Verification items for the finished model (mm, model axes). A direction names the side the tool comes from. Round coordinates to 2 decimals unless told otherwise and drop trailing zeros. Write each loop counter-clockwise with the first axis right and the second up, starting at its lowest first coordinate (ties: lowest second). Pieces come first, ordered by that corner, then holes. Notation, with made-up numbers: M -37,86 L 11,86 A36 cw 11,125 Z; hole C -19,48.5 d8. An arc over 180 degrees is marked long. One line per question, with ' | ' between items.
from build123d import *

# Parameters (mm, degrees)
F1_DEPTH = 63.5
F2_DEPTH = 25.4
F3_DEPTH = 3.3655
F6_R     = 6.35
F7_R     = 2.54
F8_R     = 2.54


with BuildPart() as f1:
    # F0 (on Front) → F1 (new body, symmetric)
    with BuildSketch(Plane.XZ):
        Polygon((-41.275, -9.525), (41.275, -9.525), (41.275, 9.525), (22.225, 9.525), (-41.275, 9.525), align=None)
    extrude(amount=F1_DEPTH, both=True)

    # F0 (on Front) → F2 (join, symmetric)
    with BuildSketch(Plane.XZ):
        with BuildLine():
            Line((22.225, 9.525), (41.275, 9.525))
            Line((41.275, 9.525), (41.275, 27.305))
            ThreePointArc((41.275, 27.305), (45.9246798487, 38.5303201513), (57.15, 43.18))
            Line((57.15, 43.18), (64.7230581194, 43.18))
            Line((64.7230581194, 43.18), (64.7230581194, 62.23))
            Line((64.7230581194, 62.23), (57.15, 62.23))
            ThreePointArc((57.15, 62.23), (32.4542956671, 52.0007043329), (22.225, 27.305))
            Line((22.225, 27.305), (22.225, 9.525))
        make_face()
    extrude(amount=F2_DEPTH, both=True)

    # F0 (on Front) → F3 (join, symmetric)
    with BuildSketch(Plane.XZ):
        with BuildLine():
            add(Edge.make_bspline(
                [(-41.275, 9.525), (-13.7296449393, 37.2954718769), (24.3855025619, 65.1646107435), (64.7230581194, 62.23)],
                knots=[0, 0, 0, 0, 118.3782300514, 118.3782300514, 118.3782300514, 118.3782300514], degree=3))
            Line((-41.275, 9.525), (22.225, 9.525))
            Line((22.225, 9.525), (22.225, 27.305))
            ThreePointArc((22.225, 27.305), (32.4542956671, 52.0007043329), (57.15, 62.23))
            Line((57.15, 62.23), (64.7230581194, 62.23))
        make_face()
    extrude(amount=F3_DEPTH, both=True)

    # F0 (on Front) → F5 (revolve)
    with BuildSketch(Plane.XZ):
        Polygon((85.725, 66.675), (85.725, 62.23), (85.725, 43.18), (85.725, 38.1), (115.5230581194, 38.1), (115.5230581194, 66.675), align=None)
    revolve(axis=Axis((85.3036269546, 0, 52.5564104319), (0, 0, -1)))

    # F6
    f6_edges = [f1.edges().sort_by_distance(p)[0] for p in [
        (-41.275, -63.5, 0),
        (41.275, -63.5, 0),
        (41.275, 63.5, 0),
        (-41.275, 63.5, 0),
    ]]
    fillet(f6_edges, radius=F6_R)

    # F7
    f7_edges = [f1.edges().sort_by_distance(p)[0] for p in [
        (64.723058, -25.4, 52.705),
    ]]
    fillet(f7_edges, radius=F7_R)

    # F8
    f8_edges = [f1.edges().sort_by_distance(p)[0] for p in [
        (64.723058, 25.4, 52.705),
    ]]
    fillet(f8_edges, radius=F8_R)


solid = f1.part
1. Tool access check on faces 1 (the face through (86, 0, 38.1)), 2 (the face through (37, -25.4, 36)), 3 (the face through (37, 25.4, 36)). Record the directions out of +Z, -Z, +X, -X, +Y, -Y that give a thin tool (end or side, any length) a straight path to the whole face; none if there is none.
Results:
face 1: -Z, +X, +Y, -Y | face 2: +Z, -X, -Y | face 3: +Z, -X, +Y
2. Thickness scan on line 1 (Z direction, x = 9.5, y = -52) (3 decimals); line 2 (Y direction, x = -17, z = 27); line 3 (Z direction, x = 85, y = -4) (3 decimals). Record the ranges inside material, lowest first.
Results:
line 1: z = -9.525 to 9.525 | line 2: y = -3.37 to 3.37 | line 3: z = 38.1 to 66.675
3. Go/stop test with flat-tipped pins: P1, Ø2, axis at x = 43, y = 7.5, coming from the +Z side; P2, Ø4, axis at y = -0.5, z = 19, coming from the -X side; P3, Ø9, axis at y = -11, z = 14.5, coming from the -X side (3 decimals); P4, Ø6, axis at x = 50.5, y = 31, coming from the +Z side. Record where each tip stops, or that it passes through.
Results:
P1: stops at z = 59.66 | P2: stops at x = -33.59 | P3: stops at x = 22.225 | P4: passes through
4. Section check C-C, the plane x = 59. Record the cut outline in (y, z) (3 decimals).
Results:
outline: M -25.4,43.18 L -14.877,43.18 L -14.877,38.1 L 14.877,38.1 L 14.877,43.18 L 25.4,43.18 L 25.4,62.23 L 14.877,62.23 L 14.877,66.675 L -14.877,66.675 L -14.877,62.23 L -25.4,62.23 Z
5. Section check A-A, the plane z = 2.5. Record the cut outline in (x, y) (3 decimals), then the cut area to 3 significant figures.
Results:
outline: M -41.275,-57.15 A6.35 ccw -34.925,-63.5 L 34.925,-63.5 A6.35 ccw 41.275,-57.15 L 41.275,57.15 A6.35 ccw 34.925,63.5 L -34.925,63.5 A6.35 ccw -41.275,57.15 Z | area: 10,400 mm2
6. Section check B-B, the plane y = 19.5. Record the cut outline in (x, z) (3 decimals), then the cut area to 3 significant figures.
Results:
outline: M -41.275,-9.525 L 41.275,-9.525 L 41.275,27.305 A15.875 cw 57.15,43.18 L 62.218,43.18 L 62.218,38.1 L 108.39,38.1 L 108.39,66.675 L 62.218,66.675 L 62.218,62.23 L 57.15,62.23 A34.925 ccw 22.225,27.305 L 22.225,9.525 L -41.275,9.525 Z | area: 4,090 mm2
7. Mould release check, pull along X, two halves, no side actions. Record for faces 4 (the face through (84.88, -0.42, 66.675)), 5 (the face through (60, -20, 43.18)), 6 (the face through (32.727, 14.229, 52.271)): pulls with the +X half, pulls with the -X half, needs draft (parallel to the pull), parting line crosses it, or undercut.
Results:
face 4: needs draft | face 5: undercut | face 6: pulls with the -X half
